Study the drawing (mm; zero at the part's minimum x, y, z) and answer. A direction names the side the tool comes from. Round coordinates to 2 decimals unless told otherwise and drop trailing zeros. Write each loop counter-clockwise with the first axis right and the second up, starting at its lowest first coordinate (ties: lowest second). Pieces come first, ordered by that corner, then holes. Notation, with made-up numbers: (-7, -1.5) - (2, -1.5) arc R13 ccw to (2, 7.5) - close; hole circle Ø9 at (10, 14). An arc over 180 degrees is marked (long way). Use one line per item in the form item = value. Start each with the question number.
1) The part is cut by section C-C, the plane x = 34. Give the vertices of the cut face in (y, z), plus the area to 3 significant figures.
2) For the marked faces 1, 2, 3 and 4, determine the directions among +Z, -Z, +X, -X, +Y, -Y from which every point of the face is accessible in a straight line to the end or side of a thin tool.
3) The part is cut by section A-A, the plane y = 54. Give the vertices of the cut face in (x, z), plus the area to 3 significant figures.
4) The part is cut by section D-D, the plane z = 14. Give the vertices of the cut face in (x, y), plus the area to 3 significant figures.
5) The part is cut by section B-B, the plane z = 53.5. Give the vertices of the cut face in (x, y).
6) Consider line 1 along Y through (x, z) = (68.5, 53); line 2 along Z through (x, y) = (56.5, 35); line 3 along Z through (x, y) = (36, 53). Determine where each line is inside the solid, lowest interval first. Write a range as from..to.
7) Each of these flat-tipped pins is pushed along its axis until it touches: pin 1 (6 mm diameter, centred on x = 46.5, z = 51, fed in from +Y); pin 2 (5 mm diameter, centred on x = 89, y = 45, fed in from +Z); pin 3 (16 mm diameter, centred on x = 50, z = 53, fed in from -Y). Where does it stop, or does it pass through?
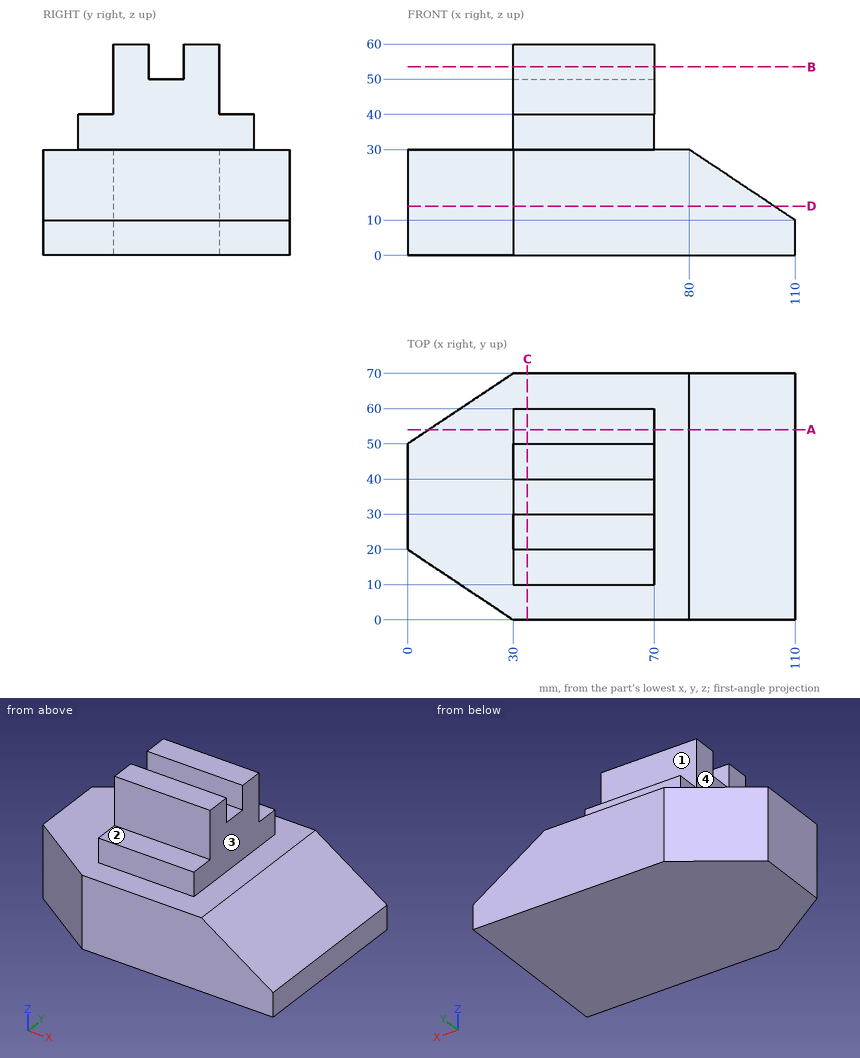
Geometry results:
q1.outline = (0, 0) - (70, 0) - (70, 30) - (60, 30) - (60, 40) - (50, 40) - (50, 60) - (40, 60) - (40, 50) - (30, 50) - (30, 60) - (20, 60) - (20, 40) - (10, 40) - (10, 30) - (0, 30) - close
q1.area = 3,100 mm2
q2.face_1 = +Z, +X, -X, +Y
q2.face_2 = +Z, +X, -X, -Y
q2.face_3 = +Z, +X, +Y, -Y
q2.face_4 = +Z, -X, +Y, -Y
q3.outline = (6, 0) - (110, 0) - (110, 10) - (80, 30) - (70, 30) - (70, 40) - (30, 40) - (30, 30) - (6, 30) - close
q3.area = 3,220 mm2
q4.outline = (0, 20) - (30, 0) - (104, 0) - (104, 70) - (30, 70) - (0, 50) - close
q4.area = 6,680 mm2
q5.outline = (30, 20) - (70, 20) - (70, 30) - (30, 30) - close; (30, 40) - (70, 40) - (70, 50) - (30, 50) - close
q6.line_1 = 20..30, 40..50
q6.line_2 = 0..50
q6.line_3 = 0..40
q7.pin_1 = 50
q7.pin_2 = 25.67
q7.pin_3 = 20
